Design review of the part built by this model. Coordinates are the model's own, in mm. Face numbers are marked on the shaded views. A direction names the side the tool comes from. Give positions to 0.01 mm unless a question says otherwise; leave off trailing zeros. Write each loop counter-clockwise with the first axis right and the second up, starting at its lowest first coordinate (ties: lowest second). Pieces come first, ordered by that corner, then holes. Notation, with made-up numbers: M 64.5,83.25 L 104.5,83.25 A23 cw 104.5,95.25 Z; hole C 72,70.25 d11. An arc over 180 degrees is marked long. One line per item, written item: value. Start each with the question number.
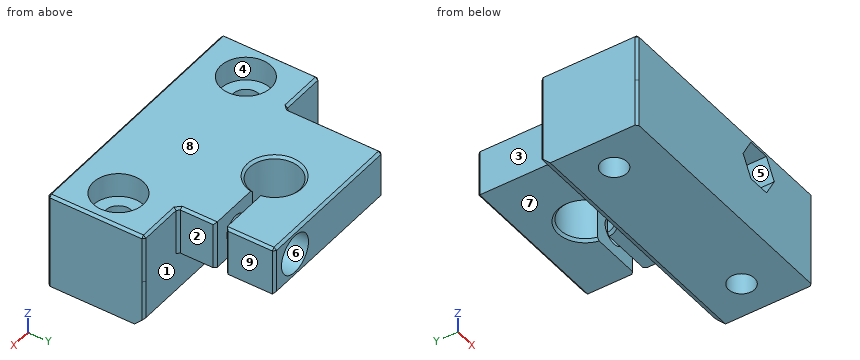
```python
from build123d import *

# Parameters (mm, degrees)
F0_R      = 5.175
F1_DEPTH  = 10
F0_R_2    = 2.675
F2_DEPTH  = 5
F3_DEPTH  = 5
F4_R      = 2.675
F5_DEPTH  = 40
F6_DEPTH  = 5
F7_R      = 4
F7_R_2    = 2.675
F8_DEPTH  = 5
F9_SIZE   = 0.5
F10_DEPTH = 10
F11_DEPTH = 10
F12_SIZE  = 0.49999
F13_SIZE  = 2


# Not quite as in the source:
# - a fillet or chamfer is up to 0.001 mm smaller than in the source, because OpenCascade refuses the exact size


with BuildPart() as f1:
    # F0 (on Top) → F1 (new body)
    with BuildSketch(Plane.XY):
        with BuildLine():
            Line((14.923914507, 11.175), (-17.076085493, 11.175))
            Line((-17.076085493, 11.175), (-17.076085493, -8.825))
            Line((-17.076085493, -8.825), (14.923914507, -8.825))
            Line((14.923914507, -8.825), (14.923914507, -1.035))
            Line((14.923914507, -1.035), (3.9943582746, -1.035))
            ThreePointArc((3.9943582746, -1.035), (-6.251085493, 0), (3.9943582746, 1.035))
            Line((3.9943582746, 1.035), (14.923914507, 1.035))
            Line((14.923914507, 1.035), (14.923914507, 11.175))
        make_face()
        Polygon((14.923914507, -8.825), (-17.076085493, -8.825), (-27.076085493, -8.825), (-27.076085493, -28.825), (-17.076085493, -28.825), (14.923914507, -28.825), (24.923914507, -28.825), (24.923914507, -8.825), align=None)
        with Locations((-19.901085493, -19.0323841524)):
            Circle(F0_R, mode=Mode.SUBTRACT)
        with Locations((17.748914507, -19.1356375643)):
            Circle(F0_R, mode=Mode.SUBTRACT)
    extrude(amount=F1_DEPTH)

    # F0 (on Top) → F2 (join)
    with BuildSketch(Plane.XY):
        with Locations((-19.901085493, -19.0323841524)):
            Circle(F0_R)
        with Locations((-19.901085493, -19.0323841524)):
            Circle(F0_R_2, mode=Mode.SUBTRACT)
    extrude(amount=F2_DEPTH)

    # F0 (on Top) → F3 (join)
    with BuildSketch(Plane.XY):
        with Locations((17.748914507, -19.1356375643)):
            Circle(F0_R)
        with Locations((17.748914507, -19.1356375643)):
            Circle(F0_R_2, mode=Mode.SUBTRACT)
    extrude(amount=F3_DEPTH)

    # F4 (on face) → F5 (cut)
    with BuildSketch(Plane.XZ.offset(28.825)):
        with Locations((8.923914507, 5)):
            Circle(F4_R)
    extrude(amount=-F5_DEPTH, mode=Mode.SUBTRACT)

    # F4 (on face) → F6 (cut)
    with BuildSketch(Plane.XZ.offset(28.825)):
        Polygon((4.3052091527, 4.9700971099), (6.6404584923, 0.9851323855), (11.2591638467, 1.0150352756), (13.5426198614, 5.0299028901), (11.2073705218, 9.0148676145), (6.5886651674, 8.9849647244), align=None)
        with Locations((8.923914507, 5)):
            Circle(F4_R, mode=Mode.SUBTRACT)
    extrude(amount=-F6_DEPTH, mode=Mode.SUBTRACT)

    # F7 (on face) → F8 (cut)
    with BuildSketch(Plane(origin=(0, 11.175, 0), x_dir=(-1, 0, 0), z_dir=(0, 1, 0))):
        with Locations((-8.923914507, 5)):
            Circle(F7_R)
        with Locations((-8.923914507, 5)):
            Circle(F7_R_2, mode=Mode.SUBTRACT)
    extrude(amount=-F8_DEPTH, mode=Mode.SUBTRACT)

    # F9
    f9_edges = [f1.edges().sort_by_distance(p)[0] for p in [
        (-27.076085, -18.825, 10),
        (-22.076085, -8.825, 10),
        (-17.076085, 1.175, 10),
        (-1.076085, 11.175, 10),
        (14.923915, 6.105, 10),
        (14.923915, -4.93, 10),
        (19.923915, -8.825, 10),
        (24.923915, -18.825, 10),
        (24.923915, -8.825, 5),
        (14.923915, -8.825, 5),
        (14.923915, -1.035, 5),
        (14.923915, 1.035, 5),
        (14.923915, 11.175, 5),
        (-17.076085, 11.175, 5),
        (-17.076085, -8.825, 5),
        (-27.076085, -8.825, 5),
        (-27.076085, -28.825, 5),
        (24.923915, -28.825, 5),
        (-6.251085, 0, 10),
        (-1.076085, -28.825, 10),
        (-6.251085, 0, 0),
        (-1.076085, 11.175, 0),
    ]]
    chamfer(f9_edges, length=F9_SIZE)

    # F0 (on Top) → F10 (join)
    with BuildSketch(Plane.XY):
        Polygon((14.923914507, -8.825), (-17.076085493, -8.825), (-27.076085493, -8.825), (-27.076085493, -28.825), (-17.076085493, -28.825), (14.923914507, -28.825), (24.923914507, -28.825), (24.923914507, -8.825), align=None)
        with Locations((-19.901085493, -19.0323841524)):
            Circle(F0_R, mode=Mode.SUBTRACT)
        with Locations((17.748914507, -19.1356375643)):
            Circle(F0_R, mode=Mode.SUBTRACT)
    extrude(amount=-F10_DEPTH)

    # F0 (on Top) → F11 (join)
    with BuildSketch(Plane.XY):
        with Locations((17.748914507, -19.1356375643)):
            Circle(F0_R)
        with Locations((17.748914507, -19.1356375643)):
            Circle(F0_R_2, mode=Mode.SUBTRACT)
        with Locations((-19.901085493, -19.0323841524)):
            Circle(F0_R)
        with Locations((-19.901085493, -19.0323841524)):
            Circle(F0_R_2, mode=Mode.SUBTRACT)
    extrude(amount=-F11_DEPTH)

    # F12 (size 0.5 in the source; OpenCascade refuses exactly that, so slightly less here)
    f12_edges = [f1.edges().sort_by_distance(p)[0] for p in [
        (24.923915, -8.825, -5),
        (-27.076085, -8.825, -5),
        (24.923915, -28.825, -5),
        (-27.076085, -28.825, -5),
    ]]
    chamfer(f12_edges, length=F12_SIZE)

    # F13
    f13_edges = [f1.edges().sort_by_distance(p)[0] for p in [
        (-1.076085, -8.825, -10),
    ]]
    chamfer(f13_edges, length=F13_SIZE)


solid = f1.part
```
Q1. The part is to be moulded in two halves that separate along Z. For the marked faces 6, 7, 8 and 9, say which applies: pulls with the +Z half, pulls with the -Z half, needs draft (parallel to the pull), parting line crosses it, or undercut.
Q2. Wall thickness on line 1 (X direction, y = 2.75, z = 5); line 2 (Y direction, x = 6, z = 2.75) (3 decimals); line 3 (X direction, y = -21.5, z = 0): over which ranges is each line inside the solid? List them lowest first. Write a range as from..to.
Q3. Take a section at B-B, the plane x = 8. State how many separate pieces and enclosed holes the cut face has, then the cut area to 3 significant figures.
Q4. Take a section at C-C, the plane z = -0.75. Give the boundary of the cut face in (x, y) (3 decimals).
Q5. For P1, Ø5, axis at y = -1.5, z = -2, coming from the -X side; P2, Ø2, axis at y = 4, z = 5.5, coming from the +X side; P3, Ø3, axis at x = 7.5, z = 4.5, coming from the -Y side (3 decimals), all flat-tipped, find the tip position at first contact; note any pin that passes through.
Q6. Take a section at D-D, the plane x = -13. Give the boundary of the cut face in (y, z) (3 decimals).
Q7. Machinability: for the marked faces 1, 2, 3, 4 and 5, which of the approach directions +Z, -Z, +X, -X, +Y, -Y give a long, thin tool a straight path to every point of the face, cutting with its end or side? Answer none if there is none.
Q8. Take a section at A-A, the plane y = 0. Give the boundary of the cut face in (x, z), then the cut area to 3 significant figures.
Results list:
1. face 6: undercut
1. face 7: pulls with the -Z half
1. face 8: pulls with the +Z half
1. face 9: needs draft
2. line 1: x = -17.08..-5.46, 3.31..6.25, 11.6..14.92
2. line 2: y = -23.825..-1.035, 1.035..6.175
2. line 3: x = -27.08..-20.93, -18.87..16.5, 19..24.92
3. separate pieces: 4
3. enclosed holes: 0
3. area: 358 mm^2
4. outline: M -27.076,-28.325 L -26.576,-28.825 L 24.424,-28.825 L 24.924,-28.325 L 24.924,-9.325 L 24.424,-8.825 L -26.576,-8.825 L -27.076,-9.325 Z; hole C -19.901,-19.032 d5.35; hole C 17.749,-19.136 d5.35
5. P1: stops at x = -17.08
5. P2: stops at x = 14.92
5. P3: stops at y = -23.825
6. outline: M -28.825,-10 L -10.825,-10 L -8.825,-8 L -8.825,0 L 10.675,0 L 11.175,0.5 L 11.175,9.5 L 10.675,10 L -28.325,10 L -28.825,9.5 Z
7. face 1: -Z, +Y
7. face 2: +Z, -Z, +X, +Y
7. face 3: +Z, -Z, -X, +Y
7. face 4: +Z
7. face 5: -Y
8. outline: M -17.08,0 L -6.75,0 L -6.25,0.5 L -6.25,9.5 L -6.75,10 L -16.58,10 L -17.08,9.5 Z
8. area: 108 mm^2
